```python
from build123d import *

# Parameters (mm, degrees)
SALIENTE_EXTRUIR1_DEPTH   = 5
SALIENTE_EXTRUIR1_2_DEPTH = 5
SALIENTE_EXTRUIR1_3_DEPTH = 5
SALIENTE_EXTRUIR1_4_DEPTH = 5
CROQUIS3_W                = 20
CROQUIS3_H                = 20
SALIENTE_EXTRUIR2_DEPTH   = 5
REDONDEO1_R               = 2
CROQUIS4_W                = 20
CROQUIS4_H                = 25
SALIENTE_EXTRUIR3_DEPTH   = 5
CORTAR_EXTRUIR1_DEPTH     = 31.822070015
CORTAR_EXTRUIR2_DEPTH     = 31.232432916


with BuildPart() as part:
    # Croquis2 → Saliente-Extruir1 (new body)
    with BuildSketch(Plane(origin=(0, 0, 0), x_dir=(1, 0, 0), z_dir=(0, 1, 0))):
        Polygon((-3.880962474, 9.7), (-4.31520152, 10), (4.31520152, 10), (3.880962474, 9.7), (3.100109842, 9.007732001), (3.100109842, 7.886854264), (5.174607071, 7.886854264), (5.174607071, 6.657084853), (2.689193029, 4.171670811), (-2.689193029, 4.171670811), (-5.174607071, 6.657084853), (-5.174607071, 7.886854264), (-3.100109842, 7.886854264), (-3.100109842, 9.007732001), align=None)
    extrude(amount=SALIENTE_EXTRUIR1_DEPTH)



with BuildPart() as body_2:
    # Croquis2 → Saliente-Extruir1 2 (new body)
    with BuildSketch(Plane(origin=(0, 0, 0), x_dir=(1, 0, 0), z_dir=(0, 1, 0))):
        Polygon((10, 4.31520152), (10, -4.31520152), (9.7, -3.880962474), (9.007732001, -3.100109842), (7.886854264, -3.100109842), (7.886854264, -5.174607071), (6.657084853, -5.174607071), (4.171670811, -2.689193029), (4.171670811, 2.689193029), (6.657084853, 5.174607071), (7.886854264, 5.174607071), (7.886854264, 3.100109842), (9.007732001, 3.100109842), (9.7, 3.880962474), align=None)
    extrude(amount=SALIENTE_EXTRUIR1_2_DEPTH)


with BuildPart() as body_3:
    # Croquis2 → Saliente-Extruir1 3 (new body)
    with BuildSketch(Plane(origin=(0, 0, 0), x_dir=(1, 0, 0), z_dir=(0, 1, 0))):
        Polygon((4.31520152, -10), (-4.31520152, -10), (-3.880962474, -9.7), (-3.100109842, -9.007732001), (-3.100109842, -7.886854264), (-5.174607071, -7.886854264), (-5.174607071, -6.657084853), (-2.689193029, -4.171670811), (2.689193029, -4.171670811), (5.174607071, -6.657084853), (5.174607071, -7.886854264), (3.100109842, -7.886854264), (3.100109842, -9.007732001), (3.880962474, -9.7), align=None)
    extrude(amount=SALIENTE_EXTRUIR1_3_DEPTH)


with BuildPart() as body_4:
    # Croquis2 → Saliente-Extruir1 4 (new body)
    with BuildSketch(Plane(origin=(0, 0, 0), x_dir=(1, 0, 0), z_dir=(0, 1, 0))):
        Polygon((-10, -4.31520152), (-10, 4.31520152), (-9.7, 3.880962474), (-9.007732001, 3.100109842), (-7.886854264, 3.100109842), (-7.886854264, 5.174607071), (-6.657084853, 5.174607071), (-4.171670811, 2.689193029), (-4.171670811, -2.689193029), (-6.657084853, -5.174607071), (-7.886854264, -5.174607071), (-7.886854264, -3.100109842), (-9.007732001, -3.100109842), (-9.7, -3.880962474), align=None)
    extrude(amount=SALIENTE_EXTRUIR1_4_DEPTH)


with BuildPart() as part_1:
    add(part.part)

    add(body_2.part)  # Saliente-Extruir2 merges body 2

    add(body_3.part)  # Saliente-Extruir2 merges body 3

    add(body_4.part)  # Saliente-Extruir2 merges body 4
    # Croquis3 → Saliente-Extruir2 (add)
    with BuildSketch(Plane(origin=(0, 5, 0), x_dir=(1, 0, 0), z_dir=(0, 1, 0))):
        Rectangle(CROQUIS3_W, CROQUIS3_H)
    extrude(amount=SALIENTE_EXTRUIR2_DEPTH)

    # Redondeo1
    redondeo1_edges = [part_1.edges().sort_by_distance(p)[0] for p in [
        (10, 10, 0),
        (0, 10, -10),
        (-10, 10, 0),
        (0, 10, 10),
    ]]
    fillet(redondeo1_edges, radius=REDONDEO1_R)

    # Croquis4 → Saliente-Extruir3 (add)
    with BuildSketch(Plane.XY.offset(10)):
        with Locations((0, -4.5)):
            Rectangle(CROQUIS4_W, CROQUIS4_H)
    extrude(amount=SALIENTE_EXTRUIR3_DEPTH)

    # Croquis5 → Cortar-Extruir1 (cut, through all)
    with BuildSketch(Plane(origin=(0, 8, 0), x_dir=(1, 0, 0), z_dir=(0, 1, 0))):
        Polygon((4.006067099, -15), (-4.006067099, -15), (-3.450123093, -13.373585697), (3.450123093, -13.373585697), align=None)
    extrude(amount=-CORTAR_EXTRUIR1_DEPTH, mode=Mode.SUBTRACT)

    # Croquis6 → Cortar-Extruir2 (cut, through all)
    with BuildSketch(Plane(origin=(10, 0, 0), x_dir=(0, 0, -1), z_dir=(1, 0, 0))):
        with BuildLine():
            Line((-15, 5.73584659), (-15, 0.367400389))
            ThreePointArc((-15, 0.367400389), (-12.315776899, 3.051623489), (-15, 5.73584659))
        make_face()
        with BuildLine():
            Line((-15, -2.26415341), (-15, -7.632599611))
            ThreePointArc((-15, -7.632599611), (-12.315776899, -4.948376511), (-15, -2.26415341))
        make_face()
        with BuildLine():
            Line((-15, -10.26415341), (-15, -15.632599611))
            ThreePointArc((-15, -15.632599611), (-12.315776899, -12.948376511), (-15, -10.26415341))
        make_face()
    extrude(amount=-CORTAR_EXTRUIR2_DEPTH, mode=Mode.SUBTRACT)


solid = part_1.part
```
Check sheet for the modelled part. Datum: model origin and axes. Units: mm. A direction names the side the tool comes from. Round coordinates to 2 decimals unless told otherwise and drop trailing zeros. Order: outer loops, then holes, each group sorted by start corner. A loop starts at its lowest first (then second) coordinate and runs counter-clockwise, first axis right, second up. Notation, with made-up numbers: (14, -25.75) -> (68, -25.75) arc R14 ccw to (68, -11.75) -> close; hole circle Ø10 at (5, -39). An arc over 180 degrees is marked (long way). One line per item, written item: value. Start each with the question number.
Q1. Cross-section at D-D (y = 2.25). Give the number of separate pieces and of enclosed holes in the cut face, and give its area (3 significant figures).
Q2. Cross-section at C-C (x = -2). Record the boundary of the cut face in (y, z), and give its area (3 significant figures).
Q3. Gauge pin test, flat ends, axial feed: pin 1 Ø1 at (x, y) = (2, -14) entering from -Z; pin 2 Ø6 at (x, y) = (-3.5, -5) entering from +Z; pin 3 Ø2.5 at (x, y) = (4.5, 2) entering from +Z; pin 4 Ø0.6 at (y, z) = (3, -7) entering from +X. Record the tip position at first contact, or that the pin passes through.
Q4. Cross-section at A-A (z = 2.25). Record the boundary of the cut face in (x, y).
Q5. Cross-section at B-B (y = -1). Record the boundary of the cut face in (x, z), and give its area (3 significant figures).
Q6. Mould release check, pull along Z, two halves, no side actions. Record for faces 4 (the face through (-7, 2, -5.175)), 5 (the face through (4.172, 2, 0)), 6 (the face through (-7, -1, 15)), 7 (the face through (-3.1, 2.5, 8.5)): pulls with the +Z half, pulls with the -Z half, needs draft (parallel to the pull), parting line crosses it, or undercut.
Q7. Thickness scan on line 1 (Z direction, x = -2.5, y = -10); line 2 (Y direction, x = 0.5, z = 0.25); line 3 (Y direction, x = 4.75, z = 7.5). Record the ranges inside material, lowest first.
Q8. Set-up check for faces 1 (the face through (-5.175, 2, -7)), 2 (the face through (0, -9, 13.374)), 3 (the face through (-7.887, 2, 4)): record each of +Z, -Z, +X, -X, +Y, -Y from which the full face is reachable in a straight line by a thin tool's end or side.
Completed:
1. separate pieces: 4
1. enclosed holes: 0
1. area: 235 mm²
2. outline: (-17, 10) -> (0, 10) -> (0, 4.17) -> (5, 4.17) -> (5, -4.17) -> (0, -4.17) -> (0, -10) -> (8, -10) arc R2 ccw to (10, -8) -> (10, 8) arc R2 ccw to (8, 10) -> (8, 13.37) -> (5.19, 13.37) arc R2.68 cw to (0.92, 13.37) -> (-2.81, 13.37) arc R2.68 cw to (-7.08, 13.37) -> (-10.81, 13.37) arc R2.68 cw to (-15.08, 13.37) -> (-17, 13.37) -> close
2. area: 231 mm²
3. pin 1: stops at z = 10
3. pin 2: stops at z = 15
3. pin 3: stops at z = 13.62
3. pin 4: stops at x = 5.17
4. outline: (-10, 0) -> (-4.17, 0) -> (-4.17, 5) -> (4.17, 5) -> (4.17, 0) -> (10, 0) -> (10, 8) arc R2 ccw to (8, 10) -> (-8, 10) arc R2 ccw to (-10, 8) -> close
5. outline: (-10, 10) -> (10, 10) -> (10, 15) -> (4.01, 15) -> (3.45, 13.37) -> (-3.45, 13.37) -> (-4.01, 15) -> (-10, 15) -> close
5. area: 87.9 mm²
6. face 4: pulls with the -Z half
6. face 5: undercut
6. face 6: pulls with the +Z half
6. face 7: undercut
7. line 1: z = 10 to 13.37
7. line 2: y = 5 to 10
7. line 3: y = 0 to 10
8. face 1: -Z, -X, -Y
8. face 2: +Z, +Y, -Y
8. face 3: -Y
